from build123d import *

# Parameters (mm, degrees)
SKETCH1_R           = 2.5
BOSS_EXTRUDE1_DEPTH = 5.08
FILLET1_R           = 5.08
FILLET2_R           = 5.08


with BuildPart() as part:
    # Sketch1 → Boss-Extrude1 (new body)
    with BuildSketch(Plane(origin=(0, 0, 0), x_dir=(1, 0, 0), z_dir=(0, 1, 0))):
        Polygon((0, 0), (0, 76.2), (25.4, 76.2), (76.2, 25.4), (76.2, 0), align=None)
        with Locations(Location((12.7, 63.5, 0), (0, 0, 270))):
            Circle(SKETCH1_R, mode=Mode.SUBTRACT)
        with Locations(Location((63.5, 12.7, 0), (0, 0, 270))):
            Circle(SKETCH1_R, mode=Mode.SUBTRACT)
        with Locations(Location((12.7, 46.99, 0), (0, 0, 270))):
            Circle(SKETCH1_R, mode=Mode.SUBTRACT)
        with Locations(Location((12.7, 30.48, 0), (0, 0, 270))):
            Circle(SKETCH1_R, mode=Mode.SUBTRACT)
        with Locations(Location((46.99, 12.7, 0), (0, 0, 270))):
            Circle(SKETCH1_R, mode=Mode.SUBTRACT)
        with Locations(Location((30.48, 12.7, 0), (0, 0, 270))):
            Circle(SKETCH1_R, mode=Mode.SUBTRACT)
        with Locations(Location((12.7, 12.7, 0), (0, 0, 270))):
            Circle(SKETCH1_R, mode=Mode.SUBTRACT)
    extrude(amount=BOSS_EXTRUDE1_DEPTH)

    # Fillet1
    fillet1_edges = [part.edges().sort_by_distance(p)[0] for p in [
        (0, 2.54, 0),
    ]]
    fillet(fillet1_edges, radius=FILLET1_R)

    # Fillet2
    fillet2_edges = [part.edges().sort_by_distance(p)[0] for p in [
        (0, 2.54, -76.2),
        (25.4, 2.54, -76.2),
        (76.2, 2.54, -25.4),
        (76.2, 2.54, 0),
    ]]
    fillet(fillet2_edges, radius=FILLET2_R)


solid = part.part
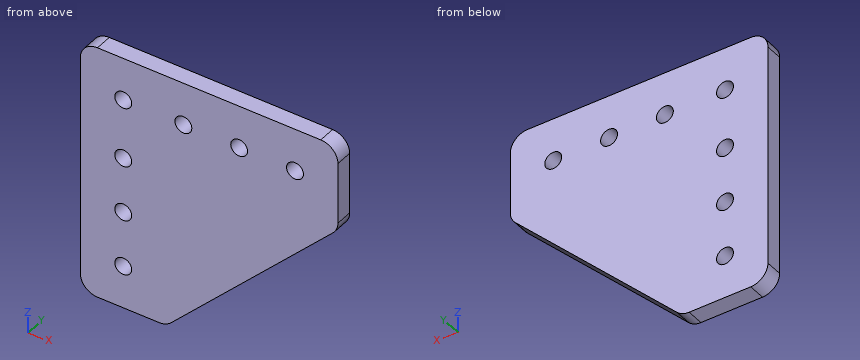
The listing builds one solid part. Answer for the finished solid, in the listing's coordinates (mm). Round coordinates to 2 decimals unless told otherwise and drop trailing zeros. Write each loop counter-clockwise with the first axis right and the second up, starting at its lowest first coordinate (ties: lowest second). Pieces come first, ordered by that corner, then holes. Notation, with made-up numbers: M 5.5,57.5 L 33.5,57.5 A12 cw 33.5,75.5 Z; hole C -12.5,11.5 d9. An arc over 180 degrees is marked long. Write each question's results on one line, items separated by ' | '. Start each with the question number.
Item 1: Find section C-C on x = 12.7. Write down the section's boundary in (y, z), and give its area (3 significant figures).
Item 2: Find section D-D on z = -12.7. Write down the section's boundary in (x, y).
Item 3: Find section B-B on x = 63.5. Write down the section's boundary in (y, z).
Item 4: Straight lines are drawn through the part: probe 1 along X at (y, z) = (3.55, -12.7); probe 2 along X at (y, z) = (1.2, -63.5); probe 3 along Z at (x, y) = (48.5, 3.7). For each, find the intervals that lie inside material, in ascending order.
Item 5: Find section A-A on z = -30.48. Write down the section's boundary in (x, y), and give its area (3 significant figures).
Item 6: Given pin 1 Ø6.5 at (x, z) = (46.99, -12.7) entering from +Y; pin 2 Ø1.5 at (x, y) = (45, 4) entering from -Z; pin 3 Ø4.5 at (x, z) = (12.7, -30.48) entering from +Y, each flat-ended and moving along its own axis, determine where each tip first touches the part or whether it passes through.
Answer block:
1) outline: M 0,-76.2 L 5.08,-76.2 L 5.08,-66 L 0,-66 Z; M 0,-61 L 5.08,-61 L 5.08,-49.49 L 0,-49.49 Z; M 0,-44.49 L 5.08,-44.49 L 5.08,-32.98 L 0,-32.98 Z; M 0,-27.98 L 5.08,-27.98 L 5.08,-15.2 L 0,-15.2 Z; M 0,-10.2 L 5.08,-10.2 L 5.08,0 L 0,0 Z | area: 285 mm²
2) outline: M 0,0 L 10.2,0 L 10.2,5.08 L 0,5.08 Z; M 15.2,0 L 27.98,0 L 27.98,5.08 L 15.2,5.08 Z; M 32.98,0 L 44.49,0 L 44.49,5.08 L 32.98,5.08 Z; M 49.49,0 L 61,0 L 61,5.08 L 49.49,5.08 Z; M 66,0 L 76.2,0 L 76.2,5.08 L 66,5.08 Z
3) outline: M 0,-38.1 L 5.08,-38.1 L 5.08,-15.2 L 0,-15.2 Z; M 0,-10.2 L 5.08,-10.2 L 5.08,0 L 0,0 Z
4) probe 1: x = 0 to 10.2, 15.2 to 27.98, 32.98 to 44.49, 49.49 to 61, 66 to 76.2 | probe 2: x = 0 to 10.2, 15.2 to 38.1 | probe 3: z = -53.1 to -14.69, -10.71 to 0
5) outline: M 0,0 L 10.2,0 L 10.2,5.08 L 0,5.08 Z; M 15.2,0 L 71.12,0 L 71.12,5.08 L 15.2,5.08 Z | area: 336 mm²
6) pin 1: stops at y = 5.08 | pin 2: stops at z = -57.35 | pin 3: passes through
